```python
from build123d import *

# Parameters (mm, degrees)
SKETCH1_R           = 6.05
BOSS_EXTRUDE1_DEPTH = 6.35
BOSS_EXTRUDE2_START = -1.1
SKETCH1_3_R         = 9.025
SKETCH1_3_R_2       = 6.05
BOSS_EXTRUDE2_DEPTH = 1.1
BOSS_EXTRUDE3_START = 6.35
SKETCH1_4_R         = 9.025
SKETCH1_4_R_2       = 6.05
BOSS_EXTRUDE3_DEPTH = 1.1
CUT_EXTRUDE1_REACH  = 17.362
SKETCH2_R           = 2.5


with BuildPart() as part:
    # Sketch1 → Boss-Extrude1 (new body)
    with BuildSketch(Plane(origin=(0, 0, 0), x_dir=(1, 0, 0), z_dir=(0, 1, 0))):
        with Locations(Location((0, 0, 0), (0, 0, 270))):
            Circle(SKETCH1_R)
    extrude(amount=BOSS_EXTRUDE1_DEPTH)

    # Sketch1_3 → Boss-Extrude2 (add)
    # profile 1 of 2: a face of its own
    with BuildSketch(Plane(origin=(0, 0, 0), x_dir=(1, 0, 0), z_dir=(0, 1, 0)).offset(BOSS_EXTRUDE2_START)):
        with Locations(Location((0, 0, 0), (0, 0, 270))):
            Circle(SKETCH1_3_R)
        with Locations(Location((0, 0, 0), (0, 0, 270))):
            Circle(SKETCH1_3_R_2, mode=Mode.SUBTRACT)
    # profile 2 of 2: a face of its own
    with BuildSketch(Plane(origin=(0, 0, 0), x_dir=(1, 0, 0), z_dir=(0, 1, 0)).offset(BOSS_EXTRUDE2_START)):
        with Locations(Location((0, 0, 0), (0, 0, 270))):
            Circle(SKETCH1_3_R_2)
    extrude(amount=BOSS_EXTRUDE2_DEPTH)

    # Sketch1_4 → Boss-Extrude3 (add)
    # profile 1 of 2: a face of its own
    with BuildSketch(Plane(origin=(0, 0, 0), x_dir=(1, 0, 0), z_dir=(0, 1, 0)).offset(BOSS_EXTRUDE3_START)):
        with Locations(Location((0, 0, 0), (0, 0, 270))):
            Circle(SKETCH1_4_R)
        with Locations(Location((0, 0, 0), (0, 0, 270))):
            Circle(SKETCH1_4_R_2, mode=Mode.SUBTRACT)
    # profile 2 of 2: a face of its own
    with BuildSketch(Plane(origin=(0, 0, 0), x_dir=(1, 0, 0), z_dir=(0, 1, 0)).offset(BOSS_EXTRUDE3_START)):
        with Locations(Location((0, 0, 0), (0, 0, 270))):
            Circle(SKETCH1_4_R_2)
    extrude(amount=BOSS_EXTRUDE3_DEPTH)

    # Sketch2 → Cut-Extrude1 (cut, up to next)
    with BuildSketch(Plane(origin=(0, 7.45, 0), x_dir=(1, 0, 0), z_dir=(0, 1, 0)), mode=Mode.PRIVATE) as cut_extrude1_sk1:
        with Locations(Location((0, 0, 0), (0, 0, 270))):
            Circle(SKETCH2_R)
    cut_extrude1_tool1 = extrude(cut_extrude1_sk1.sketch, amount=-CUT_EXTRUDE1_REACH, mode=Mode.PRIVATE) & part.part
    add(cut_extrude1_tool1.solids().sort_by_distance((0, 7.45, 0))[0], mode=Mode.SUBTRACT)


solid = part.part
```
Can you work these out from the model? Positions are in its coordinate system, mm. A direction names the side the tool comes from. Give positions to 0.01 mm unless a question says otherwise; leave off trailing zeros. Loops run counter-clockwise (first coordinate to the right, second up) from the corner with the lowest first, then second, coordinate; pieces in that order, holes last. Notation, with made-up numbers: M 46,50.25 L 96,50.25 A14 ccw 96,73.25 Z; hole C -11,84.5 d5. An arc over 180 degrees is marked long. Answer in a Markdown table with one row per item.
1. Suppose I cut it at A-A on z = 0. Write out the boundary of the cut face in (x, y) (3 decimals).
Taken from the geometry:
| item | result |
|---|---|
| outline | M -9.025,-1.1 L -2.5,-1.1 L -2.5,7.45 L -9.025,7.45 L -9.025,6.35 L -6.05,6.35 L -6.05,0 L -9.025,0 Z; M 2.5,-1.1 L 9.025,-1.1 L 9.025,0 L 6.05,0 L 6.05,6.35 L 9.025,6.35 L 9.025,7.45 L 2.5,7.45 Z |
2. Thinking about a two-plate mould opening in Y: for faces 3 (the cylindrical face through (-5.492, 6.892, -7.162)), 4 (the flat face through (-6, 6.35, 2)), 5 (the flat face through (-2, -1.1, 2)), which applies, released by +Y, released by -Y, zero draft, split by the parting line, or undercut?
Taken from the geometry:
| item | result |
|---|---|
| face 3 | zero draft |
| face 4 | undercut |
| face 5 | released by -Y |
3. If I drill on line 1 along Y through (x, z) = (-4.75, -6.25); line 2 along X through (y, z) = (2, 0); line 3 along Z through (x, y) = (-0.25, -0.5), over which ranges is the centre line in solid material (lowest first)?
Taken from the geometry:
| item | result |
|---|---|
| line 1 | y = -1.1 to 0, 6.35 to 7.45 |
| line 2 | x = -6.05 to -2.5, 2.5 to 6.05 |
| line 3 | z = -9.02 to -2.49, 2.49 to 9.02 |
4. Which directions (+Z, -Z, +X, -X, +Y, -Y) give clear straight access to the entire face, cutting with the end or side of a thin tool? Please do faces 1 (the cylindrical face through (1.82, 3.13, 5.77)), 2 (the cylindrical face through (-5.492, -0.558, -7.162)).
Taken from the geometry:
| item | result |
|---|---|
| face 1 | none |
| face 2 | +Y, -Y |
5. Suppose I cut it at D-D on z = -3.25. Write out the boundary of the cut face in (x, y).
Taken from the geometry:
| item | result |
|---|---|
| outline | M -8.42,-1.1 L 8.42,-1.1 L 8.42,0 L 5.1,0 L 5.1,6.35 L 8.42,6.35 L 8.42,7.45 L -8.42,7.45 L -8.42,6.35 L -5.1,6.35 L -5.1,0 L -8.42,0 Z |
6. Suppose I cut it at C-C on y = 6. Write out the boundary of the cut face in (x, z), plus the area to 3 significant figures.
Taken from the geometry:
| item | result |
|---|---|
| outline | C 0,0 d12.1; hole C 0,0 d5 |
| area | 95.4 mm² |
7. Suppose I cut it at B-B on x = 0. Write out the boundary of the cut face in (y, z) (3 decimals).
Taken from the geometry:
| item | result |
|---|---|
| outline | M -1.1,-9.025 L 0,-9.025 L 0,-6.05 L 6.35,-6.05 L 6.35,-9.025 L 7.45,-9.025 L 7.45,-2.5 L -1.1,-2.5 Z; M -1.1,2.5 L 7.45,2.5 L 7.45,9.025 L 6.35,9.025 L 6.35,6.05 L 0,6.05 L 0,9.025 L -1.1,9.025 Z |
